Geometry: see drawing. Coordinates: mm, zero at the bounding-box minimum. A direction names the side the tool comes from. Coordinates: 2 decimals unless noted, no trailing zeros. Write each loop counter-clockwise with the first axis right and the second up, starting at its lowest first coordinate (ties: lowest second). Pieces come first, ordered by that corner, then holes. Notation, with made-up numbers: (-38, -2) - (7, -2) arc R16 ccw to (7, 2) - close; hole circle Ø3 at (-27, -5). An arc over 180 degrees is marked (long way). Use a Markdown table: item, result. Add a question column.
Q1. Section query A-A (z = 54). Return the cut outline in (x, y), then the cut area to 3 significant figures.
Q2. Set-up query: the marked faces 1 and 2. Return all of +Z, -Z, +X, -X, +Y, -Y with unobstructed straight access to the full face (end or side cutting, diameter ignored); none if empty.
Q3. Pin query (flat end, axial travel): P1, Ø2, axis at x = 46.5, y = 20.5, coming from the -Z side. Return the tip coordinate at first contact, or that it passes through.
Q4. Mould query, pull axis X, two halves, no side actions, for the marked faces 3, 4 and 5. Classes: released by +X, released by -X, zero draft, split by the parting line, or undercut.
Q5. Section query C-C (z = 67). Return the cut outline in (x, y).
Q6. Section query D-D (x = 36.5). Return the cut outline in (y, z) (1 decimal).
Q7. Section query B-B (y = 55.5). Return the cut outline in (x, z).
Q8. Material intervals for probe 1 along X at (y, z) = (26, 72.5); probe 2 along X at (y, z) = (10, 82); probe 3 along Z at (x, y) = (10.5, 24), sorted ascending. Write a range as from..to.
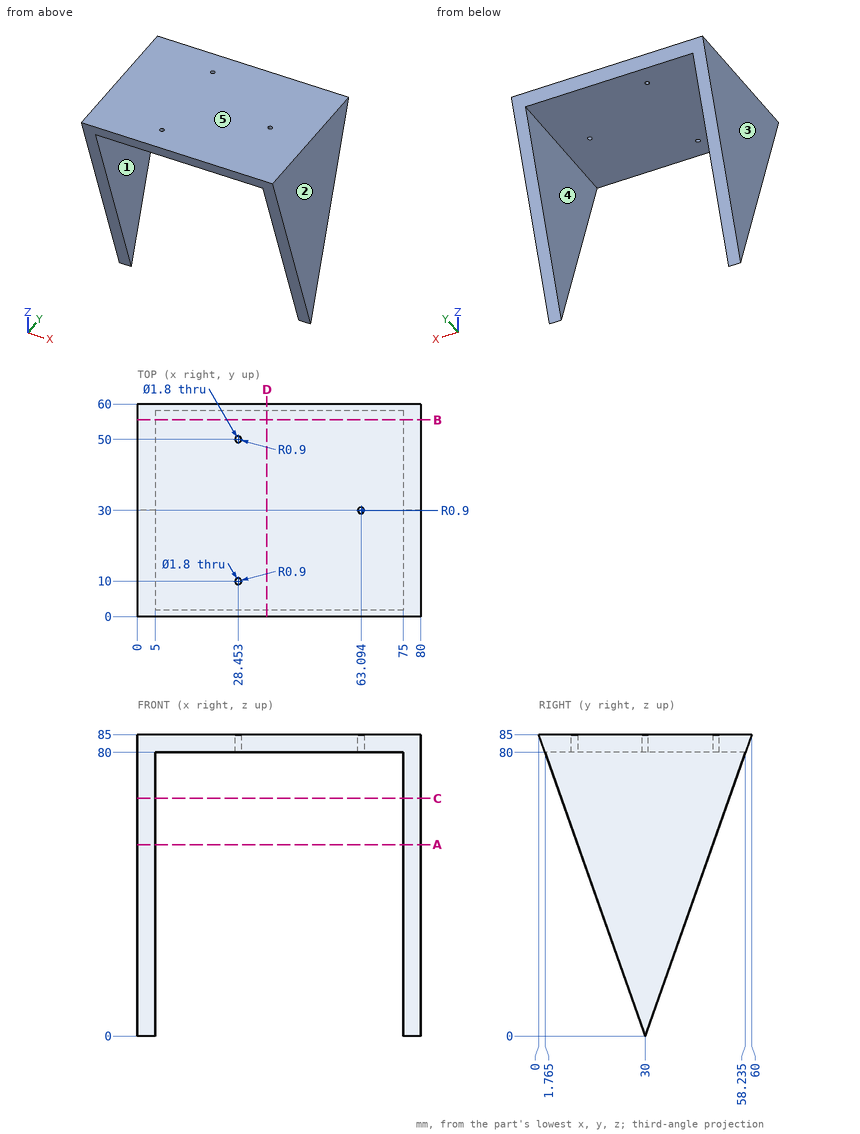
Values follow:
| question | item | result |
|---|---|---|
| 1 | outline | (0, 10.94) - (5, 10.94) - (5, 49.06) - (0, 49.06) - close; (75, 10.94) - (80, 10.94) - (80, 49.06) - (75, 49.06) - close |
| 1 | area | 381 mm2 |
| 2 | face 1 | -Z, +Y, -Y |
| 2 | face 2 | +Z, -Z, +X, +Y, -Y |
| 3 | P1 | z = 80 |
| 4 | face 3 | released by -X |
| 4 | face 4 | undercut |
| 4 | face 5 | zero draft |
| 5 | outline | (0, 6.35) - (5, 6.35) - (5, 53.65) - (0, 53.65) - close; (75, 6.35) - (80, 6.35) - (80, 53.65) - (75, 53.65) - close |
| 6 | outline | (0, 85) - (1.8, 80) - (58.2, 80) - (60, 85) - close |
| 7 | outline | (0, 72.25) - (5, 72.25) - (5, 80) - (75, 80) - (75, 72.25) - (80, 72.25) - (80, 85) - (0, 85) - close |
| 8 | probe 1 | 0..5, 75..80 |
| 8 | probe 2 | 0..27.55, 29.35..80 |
| 8 | probe 3 | 80..85 |
